from build123d import *

# Parameters (mm, degrees)
BOSS_EXTRUDE1_DEPTH = 6.35


with BuildPart() as part:
    # Sketch1 → Boss-Extrude1 (new body)
    with BuildSketch(Plane(origin=(0, 0, 0), x_dir=(1, 0, 0), z_dir=(0, 1, 0))):
        with BuildLine():
            Line((0, 0), (0, -234.95))
            ThreePointArc((0, -234.95), (-11.289784316, -252.322290845), (-31.75, -249.061111111))
            Line((-31.75, -249.061111111), (-67.13994853, -217.111852022))
            ThreePointArc((-67.13994853, -217.111852022), (-76.568587152, -201.625781937), (-75.984870047, -183.504610141))
            Line((-75.984870047, -183.504610141), (-50.8, -107.95))
            ThreePointArc((-50.8, -107.95), (-37.112138852, -45.218522559), (-37.04854536, 18.988889479))
            ThreePointArc((-37.04854536, 18.988889479), (-36.913147406, 25.420628086), (-35.166213845, 31.612059039))
            Line((-35.166213845, 31.612059039), (-20.259833627, 66.675))
            ThreePointArc((-20.259833627, 66.675), (8.490957784, 38.700189421), (19.05, 0))
            Line((19.05, 0), (0, 0))
        make_face()
    extrude(amount=BOSS_EXTRUDE1_DEPTH)


solid = part.part
For this review, take the finished solid that the model builds, in its own axes (mm). Round coordinates to 2 decimals unless told otherwise and drop trailing zeros. Order: outer loops, then holes, each group sorted by start corner. A loop starts at its lowest first (then second) coordinate and runs counter-clockwise, first axis right, second up. Notation, with made-up numbers: (28, -18.5) -> (59, -18.5) arc R11 cw to (59, -13.5) -> close; hole circle Ø8 at (-33.5, 70.5). An arc over 180 degrees is marked (long way). Write item = value, one per line. Start each with the question number.
1) To check wall thickness, follow line 1 (X direction, y = 2, z = 11.5); line 2 (X direction, y = 3, z = -3); line 3 (Z direction, x = -2, y = 1). State the ranges of each line that lie inside material, in increasing order. Write a range as from..to.
2) Take a section at C-C on x = -45. State the section outline as (y, z) points, plus the area to 3 significant figures.
3) Take a section at B-B on y = 3.25. State the section outline as (x, z) points (3 decimals), plus the area to 3 significant figures.
4) Take a section at A-A on z = 157. State the section outline as (x, y) points.
5) Insertion check: pin 1 (3 mm diameter, centred on x = -54, y = 4, fed in from +Z); pin 2 (1.9 mm diameter, centred on x = 11, y = 2, fed in from +Z); pin 3 (3 mm diameter, centred on x = 2, y = 5, fed in from -Z). Each pin has a flat end and moves straight along its axis. Give the tip position at first contact, or say it passes through.
6) The part is to be moulded in two halves that separate along Z. For faces 1 (the face through (-37.21, 3.13, 46.11)), 2 (the face through (10, 3, 0)), 3 (the face through (0, 3, 116)), 4 (the face through (-27.817, 3.131, -48.898)), say which applies: +Z half, -Z half, draft (parallel to the pull), parting line (faces both ways), or undercut.
Verdict:
q1.line_1 = -35.37..0
q1.line_2 = -35.78..18.99
q1.line_3 = -52.58..243.44
q2.outline = (0, 88.36) -> (6.35, 88.36) -> (6.35, 237.1) -> (0, 237.1) -> close
q2.area = 945 mm2
q3.outline = (-75.985, 183.505) -> (-50.8, 107.95) arc R300.832 cw to (-37.049, -18.989) arc R25.4 ccw to (-35.166, -31.612) -> (-20.26, -66.675) arc R76.2 ccw to (19.05, 0) -> (0, 0) -> (0, 234.95) arc R19.011 ccw to (-31.75, 249.061) -> (-67.14, 217.112) arc R31.75 ccw to start
q3.area = 15,900 mm2
q4.outline = (-67.15, 0) -> (0, 0) -> (0, 6.35) -> (-67.15, 6.35) -> close
q5.pin_1 = 230.33
q5.pin_2 = 0
q5.pin_3 = -49.83
q6.face_1 = undercut
q6.face_2 = +Z half
q6.face_3 = draft
q6.face_4 = -Z half
